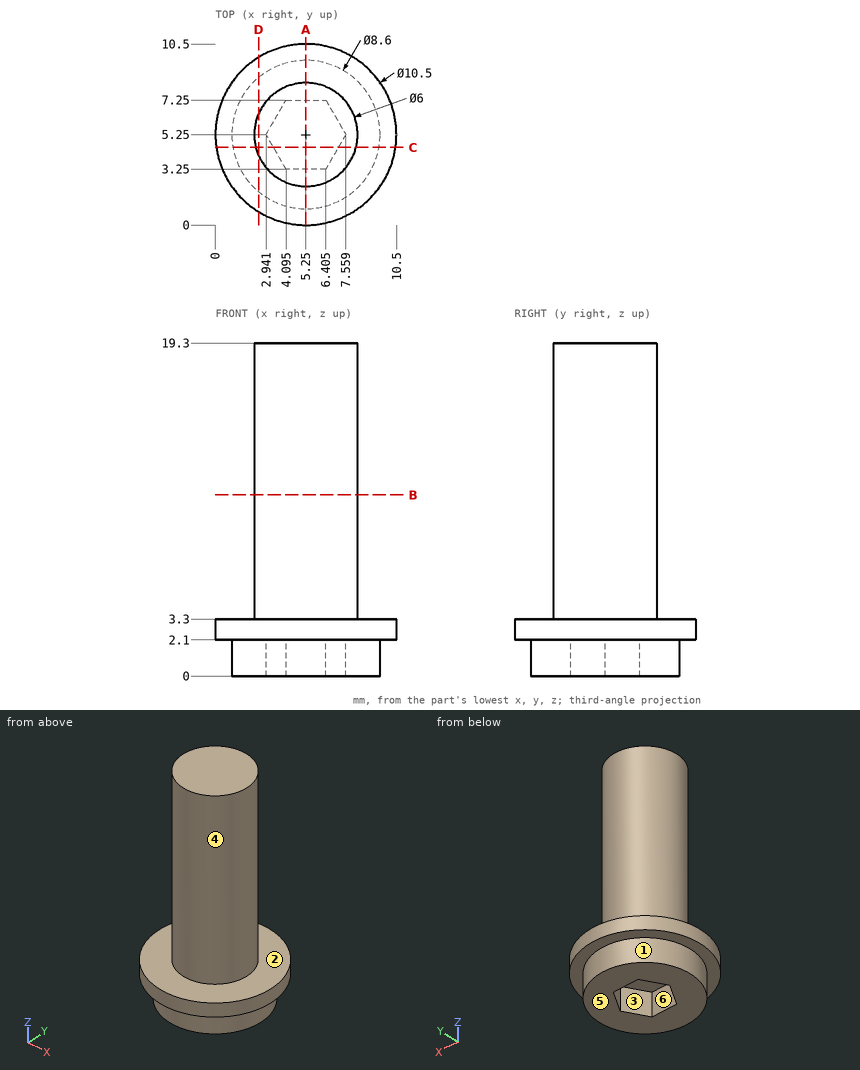
Study the drawing (mm; zero at the part's minimum x, y, z) and answer. A direction names the side the tool comes from. Give positions to 0.01 mm unless a question says otherwise; leave off trailing zeros. Write each loop counter-clockwise with the first axis right and the second up, starting at its lowest first coordinate (ties: lowest second). Pieces come first, ordered by that corner, then holes. Notation, with made-up numbers: (-14, -12) - (5, -12) arc R32 cw to (5, 23) - close; hole circle Ø7 at (45, 36.5). An arc over 180 degrees is marked (long way). Use CSV: the item, a comma, the result in double quotes. Start each with the question number.
(1) Find section B-B (z = 10.5). Give the vertices of the cut face in (x, y), plus the area to 3 significant figures.
(2) Consider line 1 along Z through (x, y) = (7.5, 2.25); line 2 along Z through (x, y) = (3.25, 9.25); line 3 along X through (y, z) = (5.75, 18). Determine where each line is inside the solid, lowest interval first.
(3) Find section C-C (y = 4.5). Give the vertices of the cut face in (x, z) (1 decimal), plus the area to 3 significant figures.
(4) For the marked faces 4, 5 and 6, determine the directions among +Z, -Z, +X, -X, +Y, -Y from which every point of the face is accessible in a straight line to the end or side of a thin tool.
(5) Determine the mould class of the marked faces 1, 2 and 3 for opening direction Y: +Y half, -Y half, draft (parallel to the pull), parting line (faces both ways), or undercut.
(6) Given P1, Ø6, axis at y = 3, z = 7, coming from the -X side; P2, Ø4, axis at y = 2.5, z = 9.5, coming from the +X side (1 decimal); P3, Ø0.6, axis at x = 5.5, z = 1, coming from the +Y side, each flat-ended and moving along its own axis, determine where each tip first touches the part or whether it passes through.
(7) Find section A-A (x = 5.25). Give the vertices of the cut face in (y, z), plus the area to 3 significant figures.
(8) Find section D-D (x = 2.5). Give the vertices of the cut face in (y, z) (1 decimal).
Findings below:
1,outline,"circle Ø6 at (5.25, 5.25)"
1,area,"28.3 mm2"
2,line 1,"0 to 3.3"
2,line 2,"2.1 to 3.3"
2,line 3,"2.29 to 8.21"
3,outline,"(0.1, 2.1) - (1, 2.1) - (1, 0) - (3.4, 0) - (3.4, 2.1) - (7.1, 2.1) - (7.1, 0) - (9.5, 0) - (9.5, 2.1) - (10.4, 2.1) - (10.4, 3.3) - (8.2, 3.3) - (8.2, 19.3) - (2.3, 19.3) - (2.3, 3.3) - (0.1, 3.3) - close"
3,area,"115 mm2"
4,face 4,"+Z"
4,face 5,"-Z, +X, -X, +Y, -Y"
4,face 6,"-Z"
5,face 1,"parting line"
5,face 2,"draft"
5,face 3,"undercut"
6,P1,"x = 2.25"
6,P2,"x = 8.2"
6,P3,"y = 9.55"
7,outline,"(0, 2.1) - (0.95, 2.1) - (0.95, 0) - (3.25, 0) - (3.25, 2.1) - (7.25, 2.1) - (7.25, 0) - (9.55, 0) - (9.55, 2.1) - (10.5, 2.1) - (10.5, 3.3) - (8.25, 3.3) - (8.25, 19.3) - (2.25, 19.3) - (2.25, 3.3) - (0, 3.3) - close"
7,area,"118 mm2"
8,outline,"(0.8, 2.1) - (1.9, 2.1) - (1.9, 0) - (8.6, 0) - (8.6, 2.1) - (9.7, 2.1) - (9.7, 3.3) - (6.4, 3.3) - (6.4, 19.3) - (4.1, 19.3) - (4.1, 3.3) - (0.8, 3.3) - close"
